from build123d import *

# Parameters (mm, degrees)
F1_DEPTH       = 15
F3_D           = 4
F3_DEPTH       = 12
F3_CSINK_D     = 8.2
F3_CSINK_ANGLE = 90
F3_TIP         = 1.2017212381


with BuildPart() as f1:
    # F0 (on Top) → F1 (new body)
    with BuildSketch(Plane.XY):
        with BuildLine():
            ThreePointArc((3, -15.638494173), (3.5277661319, -13.9390649449), (4.9253731343, -12.8375698435))
            ThreePointArc((4.9253731343, -12.8375698435), (0, 13.75), (-4.9253731343, -12.8375698435))
            ThreePointArc((-4.9253731343, -12.8375698435), (-3.5277661319, -13.9390649449), (-3, -15.638494173))
            Line((-3, -15.638494173), (-3, -33))
            ThreePointArc((-3, -33), (-3.2928932188, -33.7071067812), (-4, -34))
            Line((-4, -34), (-24, -34))
            ThreePointArc((-24, -34), (-24.7071067812, -34.2928932188), (-25, -35))
            Line((-25, -35), (-25, -39))
            ThreePointArc((-25, -39), (-24.7071067812, -39.7071067812), (-24, -40))
            Line((-24, -40), (24, -40))
            ThreePointArc((24, -40), (24.7071067812, -39.7071067812), (25, -39))
            Line((25, -39), (25, -35))
            ThreePointArc((25, -35), (24.7071067812, -34.2928932188), (24, -34))
            Line((24, -34), (4, -34))
            ThreePointArc((4, -34), (3.2928932188, -33.7071067812), (3, -33))
            Line((3, -33), (3, -15.638494173))
        make_face()
        with BuildLine():
            ThreePointArc((-3.8543283582, -10.0459819285), (0, 10.76), (3.8543283582, -10.0459819285))
            ThreePointArc((3.8543283582, -10.0459819285), (1.0637730434, -12.2453004808), (0.01, -15.638494173))
            Line((0.01, -15.638494173), (0.01, -33))
            ThreePointArc((0.01, -33), (1.1786439431, -35.8213560569), (4, -36.99))
            Line((4, -36.99), (22.01, -36.99))
            Line((22.01, -36.99), (22.01, -37.01))
            Line((22.01, -37.01), (-22.01, -37.01))
            Line((-22.01, -37.01), (-22.01, -36.99))
            Line((-22.01, -36.99), (-4, -36.99))
            ThreePointArc((-4, -36.99), (-1.1786439431, -35.8213560569), (-0.01, -33))
            Line((-0.01, -33), (-0.01, -15.638494173))
            ThreePointArc((-0.01, -15.638494173), (-1.0637730434, -12.2453004808), (-3.8543283582, -10.0459819285))
        make_face(mode=Mode.SUBTRACT)
        with BuildLine():
            ThreePointArc((4, -36.99), (1.1786439431, -35.8213560569), (0.01, -33))
            Line((0.01, -33), (-0.01, -33))
            ThreePointArc((-0.01, -33), (-1.1786439431, -35.8213560569), (-4, -36.99))
            Line((-4, -36.99), (-22.01, -36.99))
            Line((-22.01, -36.99), (-22.01, -37.01))
            Line((-22.01, -37.01), (22.01, -37.01))
            Line((22.01, -37.01), (22.01, -36.99))
            Line((22.01, -36.99), (4, -36.99))
        make_face()
    extrude(amount=F1_DEPTH)

    # F3
    with Locations(Plane(origin=(0, -34, 0), x_dir=(-1, 0, 0), z_dir=(0, 1, 0))):
        with Locations((-17.5, 7.5), (17.5, 7.5)):
            CounterSinkHole(F3_D / 2, F3_CSINK_D / 2, depth=F3_DEPTH, counter_sink_angle=F3_CSINK_ANGLE)
            with Locations((0, 0, -(F3_DEPTH + F3_TIP / 2))):  # 118° drill point
                Cone(0, F3_D / 2, F3_TIP, mode=Mode.SUBTRACT)


solid = f1.part
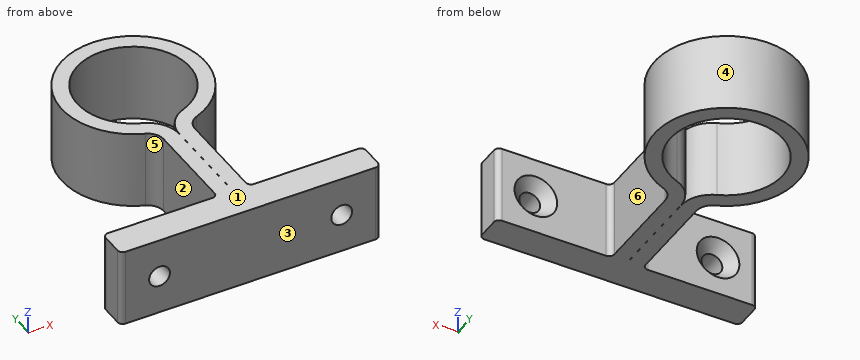
Input: part model. Units: mm. Frame: model coordinates. Face numbers are marked on the shaded views. A direction names the side the tool comes from. Round coordinates to 2 decimals unless told otherwise and drop trailing zeros. Order: outer loops, then holes, each group sorted by start corner. A loop starts at its lowest first (then second) coordinate and runs counter-clockwise, first axis right, second up. Notation, with made-up numbers: (15, -39) - (32, -39) arc R21 cw to (32, -10) - close; hole circle Ø1 at (4.5, 72). An arc over 180 degrees is marked (long way). Answer as a JSON object with one key per item and string values. Group by question number.
(1) Cut plane C-C (y = 0). Return loops of the section in (x, z).
(2) Material intervals for probe 1 along X at (y, z) = (-36.85, 7.5); probe 2 along Z at (x, y) = (17.5, -37.85); probe 3 along Y at (x, z) = (6, 8.25), sorted ascending. Write a range as from..to.
(3) Draft query along Y for the marked faces 1, 2 and 3. Return one class per face: released by +Y, released by -Y, zero draft, split by the parting line, or undercut.
(4) Pin query (flat end, axial travel): P1, Ø8, axis at y = -14.5, z = 7, coming from the -X side; P2, Ø6, axis at x = -8.5, y = 5.5, coming from the +Z side; P3, Ø5, axis at x = -17.5, z = 7.5, coming from the +Y side; P4, Ø6, axis at x = -12, z = 7, coming from the +Y side. Return the tip coordinate at first contact, or that it passes through.
(5) Cut plane D-D (y = -15). Return loops of the section in (x, z), then the cut area to 3 significant figures.
(6) Reachability of the marked faces 4, 5 and 6 from +Z, -Z, +X, -X, +Y, -Y: full face, straight path, thin tool, end or side. Return the list, or none.
(7) Cut plane A-A (z = 7.5). Count the separate pieces of the cut face and the enclosed holes in it, then the cut area to 3 significant figures.
(8) Cut plane B-B (x = -17.5). Return loops of the section in (y, z), then the cut area to 3 significant figures.
Here are the results:
{
 "1": {"outline": "(-13.75, 0) - (-10.76, 0) - (-10.76, 15) - (-13.75, 15) - close; (10.76, 0) - (13.75, 0) - (13.75, 15) - (10.76, 15) - close"},
 "2": {"probe 1": "x = -25..-19.5, -15.5..15.5, 19.5..25", "probe 2": "z = 0..5.5, 9.5..15", "probe 3": "y = -40..-34, -12.37..-8.93, 8.93..12.37"},
 "3": {"face 1": "zero draft", "face 2": "undercut", "face 3": "released by -Y"},
 "4": {"P1": "stops at x = -8.88", "P2": "stops at z = 15", "P3": "stops at y = -35.6", "P4": "stops at y = 10.4"},
 "5": {"outline": "(-3.07, 0) - (-0.04, 0) - (-0.04, 15) - (-3.07, 15) - close; (0.04, 0) - (3.07, 0) - (3.07, 15) - (0.04, 15) - close", "area": "90.7 mm^2"},
 "6": {"face 4": "+Z, -Z", "face 5": "+Z, -Z, -X", "face 6": "+Z, -Z, +X"},
 "7": {"separate pieces": "3", "enclosed holes": "1", "area": "588 mm^2"},
 "8": {"outline": "(-40, 0) - (-34, 0) - (-34, 3.4) - (-36.1, 5.5) - (-40, 5.5) - close; (-40, 9.5) - (-36.1, 9.5) - (-34, 11.6) - (-34, 15) - (-40, 15) - close", "area": "61.6 mm^2"}
}
